from build123d import *

# Parameters (mm, degrees)
F1_DEPTH = 10
F3_DEPTH = 6.25
F4_W     = 1.5
F4_H     = 11.5
F5_DEPTH = 10


with BuildPart() as f1:
    # F0 (on Right) → F1 (new body, symmetric)
    with BuildSketch(Plane.YZ):
        Polygon((-25, 0), (0, 0), (0, 60), (-10, 60), (-10, 12), (-25, 12), align=None)
    extrude(amount=F1_DEPTH, both=True)

    # F2 (on Right) → F3 (cut, symmetric)
    with BuildSketch(Plane.YZ):
        Polygon((-2.221825, 49.556349), (-10, 57.334524), (-10, 49.556349), (-6.110913, 45.667262), align=None)
        Polygon((-2.221825, 34.778175), (-10, 42.556349), (-10, 34.778175), (-6.110913, 30.889087), align=None)
        Polygon((-2.221825, 20), (-10, 27.778175), (-10, 20), (-6.110913, 16.110913), align=None)
    extrude(amount=F3_DEPTH, both=True, mode=Mode.SUBTRACT)

    # F4 (on face) → F5 (cut)
    with BuildSketch(Plane.XY.offset(12)):
        with Locations((-6.45, -17.5)):
            Rectangle(F4_W, F4_H)
        with Locations((-2.15, -17.5)):
            Rectangle(F4_W, F4_H)
        with Locations((2.15, -17.5)):
            Rectangle(F4_W, F4_H)
        with Locations((6.45, -17.5)):
            Rectangle(F4_W, F4_H)
    extrude(amount=-F5_DEPTH, mode=Mode.SUBTRACT)


solid = f1.part
Work out the finished part from the listing and answer in its coordinate system (mm). A direction names the side the tool comes from. Give positions to 0.01 mm unless a question says otherwise; leave off trailing zeros. Write each loop counter-clockwise with the first axis right and the second up, starting at its lowest first coordinate (ties: lowest second). Pieces come first, ordered by that corner, then holes.
Q1. Straight lines are drawn through the part: L1, parallel to X at y = -5.75, z = 48.5; L2, parallel to X at y = -19.25, z = 10.5; L3, parallel to Z at x = -1, y = -2.5. For each, find the intervals that lie inside material, in ascending order.
Answer:
L1: x = -10 to -6.25, 6.25 to 10
L2: x = -10 to -7.2, -5.7 to -2.9, -1.4 to 1.4, 2.9 to 5.7, 7.2 to 10
L3: z = 0 to 19.72, 20.28 to 34.5, 35.06 to 49.28, 49.83 to 60
Q2. Given pin 1 (1.6 mm diameter, centred on x = -2, y = -18.5, fed in from +Z); pin 2 (10 mm diameter, centred on y = -18, z = 39.5, fed in from -X); pin 3 (3 mm diameter, centred on x = -1, z = 18, fed in from -Y), each flat-ended and moving along its own axis, determine where each tip first touches the part or whether it passes through.
Answer:
pin 1: stops at z = 12
pin 2: passes through
pin 3: stops at y = -10
Q3. A tool of negligible diameter and unlimited length cuts with its end or side. For faces 5 (the face through (0.09, -4.19, 18.03)), 6 (the face through (7.2, -18, 7)), 7 (the face through (-0.088, -6.056, 53.391)), 8 (the face through (10, -7, 24)), from which of +Z, -Z, +X, -X, +Y, -Y can it reach the whole face along a straight path? Write none if from no direction.
Answer:
face 5: none
face 6: +Z
face 7: -Y
face 8: +Z, -Z, +X, +Y, -Y
Q4. For a pull along Y with two mould halves and no side action, classify faces 1 (the face through (0, -5, 60)), 2 (the face through (0, -25, 6)), 3 (the face through (-0.088, -4.194, 47.585)), 4 (the face through (-0.09, -8.08, 32.86)) as released by +Y, released by -Y, zero draft, split by the parting line, or undercut.
Answer:
face 1: zero draft
face 2: released by -Y
face 3: undercut
face 4: undercut
Q5. The part is cut by section A-A on y = -13.75. Give the vertices of the cut face in (x, z).
Answer:
outline: (-10, 0) - (10, 0) - (10, 12) - (7.2, 12) - (7.2, 2) - (5.7, 2) - (5.7, 12) - (2.9, 12) - (2.9, 2) - (1.4, 2) - (1.4, 12) - (-1.4, 12) - (-1.4, 2) - (-2.9, 2) - (-2.9, 12) - (-5.7, 12) - (-5.7, 2) - (-7.2, 2) - (-7.2, 12) - (-10, 12) - close
Q6. The part is cut by section D-D on y = -4.5. Give the vertices of the cut face in (x, z).
Answer:
outline: (-10, 0) - (10, 0) - (10, 60) - (-10, 60) - close; hole (-6.25, 17.72) - (6.25, 17.72) - (6.25, 22.28) - (-6.25, 22.28) - close; hole (-6.25, 32.5) - (6.25, 32.5) - (6.25, 37.06) - (-6.25, 37.06) - close; hole (-6.25, 47.28) - (6.25, 47.28) - (6.25, 51.83) - (-6.25, 51.83) - close
Q7. The part is cut by section C-C on x = 3.5. Give the vertices of the cut face in (y, z).
Answer:
outline: (-25, 0) - (0, 0) - (0, 60) - (-10, 60) - (-10, 57.33) - (-2.22, 49.56) - (-6.11, 45.67) - (-10, 49.56) - (-10, 42.56) - (-2.22, 34.78) - (-6.11, 30.89) - (-10, 34.78) - (-10, 27.78) - (-2.22, 20) - (-6.11, 16.11) - (-10, 20) - (-10, 12) - (-25, 12) - close
Q8. The part is cut by section B-B on z = 47. Give the vertices of the cut face in (x, y), and give its area (3 significant figures).
Answer:
outline: (-10, -10) - (10, -10) - (10, 0) - (-10, 0) - close; hole (-6.25, -7.44) - (6.25, -7.44) - (6.25, -4.78) - (-6.25, -4.78) - close
area: 167 mm2
